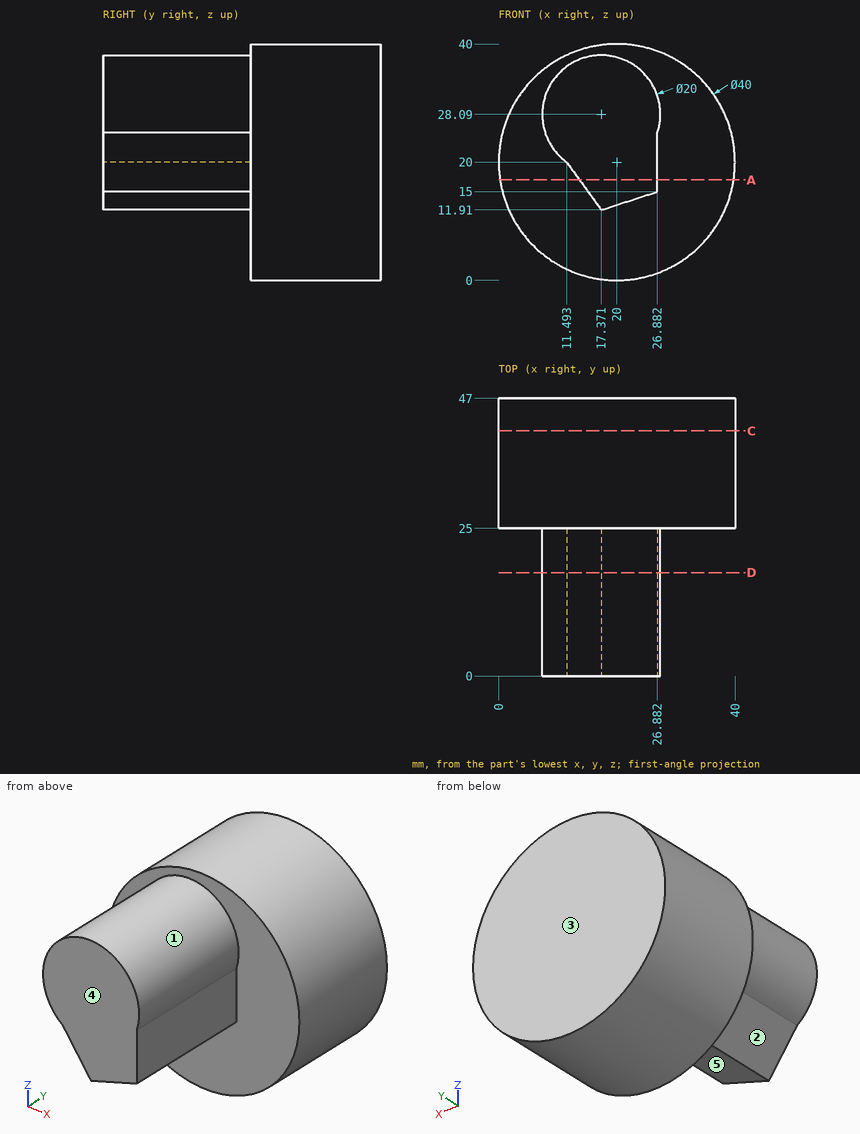
The drawing under review shows one solid part. Ordinate dimensions are in mm from its lowest x, y, z. A direction names the side the tool comes from. Give positions to 0.01 mm unless a question says otherwise; leave off trailing zeros. Write each loop counter-clockwise with the first axis right and the second up, starting at its lowest first coordinate (ties: lowest second). Pieces come first, ordered by that corner, then holes. Notation, with made-up numbers: (52, 60.25) -> (59, 60.25) arc R14 ccw to (59, 76.25) -> close; hole circle Ø3 at (-8.5, 35.5). An arc over 180 degrees is marked (long way). Use CSV: the item, a comma, the result in double quotes.
Q1. For P1, Ø10, axis at y = 29.5, z = 14, coming from the +X side (1 decimal); P2, Ø3, axis at y = 21.5, z = 28.5, coming from the -X side; P3, Ø11, axis at y = 10, z = 22.5, coming from the +X side, all flat-tipped, find the tip position at first contact; note any pin that passes through.
Conclusion:
P1,"x = 40"
P2,"x = 7.37"
P3,"x = 27.37"
Q2. Take a section at D-D, the plane y = 17.5. Write out the cut boundary in (x, z), then the cut area to 3 significant figures.
Conclusion:
outline,"(11.49, 20) -> (17.37, 11.91) -> (26.88, 15) -> (26.88, 25) arc R10 ccw (long way) to start"
area,"392 mm2"
Q3. Take a section at C-C, the plane y = 41.5. Write out the cut boundary in (x, z), then the cut area to 3 significant figures.
Conclusion:
outline,"circle Ø40 at (20, 20)"
area,"1,260 mm2"
Q4. Tool access review of the marked faces 1, 2, 3, 4 and 5: name each direction out of +Z, -Z, +X, -X, +Y, -Y from which nothing blocks a thin tool from reaching the whole face with its end or side.
Conclusion:
face 1,"-Y"
face 2,"-Z, -X, -Y"
face 3,"+Z, -Z, +X, -X, +Y"
face 4,"+Z, -Z, +X, -X, -Y"
face 5,"-Z, +X, -Y"
Q5. To check wall thickness, follow probe 1 along Y at (x, z) = (34, 28); probe 2 along Z at (x, y) = (20.5, 26.5); probe 3 along X at (y, z) = (36, 15) (1 decimal). State the ranges of each line that lie inside material, in increasing order. Write a range as [from, to].
Conclusion:
probe 1,"[25, 47]"
probe 2,"[0.01, 39.99]"
probe 3,"[0.6, 39.4]"
Q6. Take a section at A-A, the plane z = 17. Write out the cut boundary in (x, y), then the cut area to 3 significant figures.
Conclusion:
outline,"(0.23, 25) -> (13.67, 25) -> (13.67, 0) -> (26.88, 0) -> (26.88, 25) -> (39.77, 25) -> (39.77, 47) -> (0.23, 47) -> close"
area,"1,200 mm2"
